Geometry: final body of the model. Coordinates: model frame, mm. A direction names the side the tool comes from. Round coordinates to 2 decimals unless told otherwise and drop trailing zeros. Loops run counter-clockwise (first coordinate to the right, second up) from the corner with the lowest first, then second, coordinate; pieces in that order, holes last. Notation, with made-up numbers: M -6.5,41.5 L 37.5,41.5 A18 ccw 37.5,61.5 Z; hole C -33.75,19 d5. An arc over 180 degrees is marked long. Answer as a JSON object with one key per item and string values.
```python
from build123d import *

# Parameters (mm, degrees)
SKETCH1_R             = 25
BOSS_EXTRUDE1_DEPTH   = 8
CUT_EXTRUDE1_DEPTH    = 2
CUT_EXTRUDE2_DEPTH    = 36.860842154
M3X0_5_TAPPED_HOLE1_D = 2.5
CUT_EXTRUDE3_DEPTH    = 37.249137921
SKETCH7_W             = 20
SKETCH7_H             = 6
CUT_EXTRUDE4_DEPTH    = 37.249137921
FILLET1_R             = 1.5


with BuildPart() as part:
    # Sketch1 → Boss-Extrude1 (new body)
    with BuildSketch(Plane.XY):
        Circle(SKETCH1_R)
    extrude(amount=-BOSS_EXTRUDE1_DEPTH)

    # Sketch2 → Cut-Extrude1 (cut)
    with BuildSketch(Plane.XY):
        with BuildLine():
            Line((-17.5, 12.5), (17.5, 12.5))
            ThreePointArc((17.5, 12.5), (19.267766953, 11.767766953), (20, 10))
            Line((20, 10), (20, -10))
            ThreePointArc((20, -10), (19.267766953, -11.767766953), (17.5, -12.5))
            Line((17.5, -12.5), (-17.5, -12.5))
            ThreePointArc((-17.5, -12.5), (-19.267766953, -11.767766953), (-20, -10))
            Line((-20, -10), (-20, 10))
            ThreePointArc((-20, 10), (-19.267766953, 11.767766953), (-17.5, 12.5))
        make_face()
    extrude(amount=-CUT_EXTRUDE1_DEPTH, mode=Mode.SUBTRACT)

    # Sketch3 → Cut-Extrude2 (cut, through all)
    with BuildSketch(Plane.XY.offset(-2)):
        with BuildLine():
            Line((-7.5, 5), (7.5, 5))
            ThreePointArc((7.5, 5), (12.5, 0), (7.5, -5))
            Line((7.5, -5), (-7.5, -5))
            ThreePointArc((-7.5, -5), (-12.5, 0), (-7.5, 5))
        make_face()
    extrude(amount=-CUT_EXTRUDE2_DEPTH, mode=Mode.SUBTRACT)

    # M3x0.5 Tapped Hole1 (through all)
    with Locations(Plane.XY.offset(-2)):
        with Locations((16, 8.5), (-16, 8.5), (-16, -8.5), (16, -8.5)):
            Hole(M3X0_5_TAPPED_HOLE1_D / 2)

    # Sketch6 → Cut-Extrude3 (cut, through all)
    with BuildSketch(Plane.XY):
        with BuildLine():
            Line((6, 21.75), (-6, 21.75))
            ThreePointArc((-6, 21.75), (-7.060660172, 21.310660172), (-7.5, 20.25))
            Line((-7.5, 20.25), (-7.5, 15.75))
            ThreePointArc((-7.5, 15.75), (-7.060660172, 14.689339828), (-6, 14.25))
            Line((-6, 14.25), (6, 14.25))
            ThreePointArc((6, 14.25), (7.060660172, 14.689339828), (7.5, 15.75))
            Line((7.5, 15.75), (7.5, 20.25))
            ThreePointArc((7.5, 20.25), (7.060660172, 21.310660172), (6, 21.75))
        make_face()
    extrude(amount=-CUT_EXTRUDE3_DEPTH, mode=Mode.SUBTRACT)

    # Sketch7 → Cut-Extrude4 (cut, through all)
    with BuildSketch(Plane.XY):
        with Locations((0, -18)):
            Rectangle(SKETCH7_W, SKETCH7_H)
    extrude(amount=-CUT_EXTRUDE4_DEPTH, mode=Mode.SUBTRACT)

    # Fillet1
    fillet1_edges = [part.edges().sort_by_distance(p)[0] for p in [
        (10, -15, -4),
        (10, -21, -4),
        (-10, -21, -4),
        (-10, -15, -4),
    ]]
    fillet(fillet1_edges, radius=FILLET1_R)


solid = part.part
```
1) Cut plane A-A on y = 0. Return the cut outline in (x, z).
Geometry results:
{"outline": "M -25,-8 L -12.5,-8 L -12.5,-2 L -20,-2 L -20,0 L -25,0 Z; M 12.5,-8 L 25,-8 L 25,0 L 20,0 L 20,-2 L 12.5,-2 Z"}
2) Set-up query: faces 3 (the face through (20, 0, -1)), 4 (the face through (-0.3, -5.2, -8)), 5 (the face through (0, 5, -5)). Return all of +Z, -Z, +X, -X, +Y, -Y with unobstructed straight access to the full face (end or side cutting, diameter ignored); none if empty.
Geometry results:
{"face 3": "+Z", "face 4": "-Z, +X, -X, +Y, -Y", "face 5": "+Z, -Z"}
3) Pull-direction query (X, two-part tool) for faces 1 (the face through (10, -18, -4)), 2 (the face through (0, 13, 0)); classes: +X half, -X half, draft (parallel to the pull), parting line (faces both ways), or undercut.
Geometry results:
{"face 1": "undercut", "face 2": "draft"}
4) Line query: probe 1 along Y at (x, z) = (-2.5, -1.5); probe 2 along Z at (x, y) = (0, -7.5); probe 3 along Y at (x, z) = (8.5, -0.75). Output: solid intervals per line, ascending.
Geometry results:
{"probe 1": "-24.87 to -21, -15 to -12.5, 12.5 to 14.25, 21.75 to 24.87", "probe 2": "-8 to -2", "probe 3": "-23.51 to -21, -15 to -12.5, 12.5 to 23.51"}
5) First-contact query: pin 1 (1 mm diameter, centred on x = 3, z = -1.5, fed in from -Y); pin 2 (4 mm diameter, centred on x = -2, z = -4.5, fed in from -Y); pin 3 (2 mm diameter, centred on y = 13.5, z = -4.5, fed in from +X). Flat tips, straight axial feed; report the tip coordinate or a pass-through.
Geometry results:
{"pin 1": "y = -24.87", "pin 2": "y = -25", "pin 3": "x = 21.65"}
6) Cut plane B-B on z = -4.5. Return the cut outline in (x, y), and give its area (3 significant figures).
Geometry results:
{"outline": "C 0,0 d50; hole C -16,-8.5 d2.5; hole C -16,8.5 d2.5; hole M -10,-19.5 A1.5 ccw -8.5,-21 L 8.5,-21 A1.5 ccw 10,-19.5 L 10,-16.5 A1.5 ccw 8.5,-15 L -8.5,-15 A1.5 ccw -10,-16.5 Z; hole M -7.5,-5 L 7.5,-5 A5 ccw 7.5,5 L -7.5,5 A5 ccw Z; hole M -7.5,15.75 A1.5 ccw -6,14.25 L 6,14.25 A1.5 ccw 7.5,15.75 L 7.5,20.25 A1.5 ccw 6,21.75 L -6,21.75 A1.5 ccw -7.5,20.25 Z; hole C 16,-8.5 d2.5; hole C 16,8.5 d2.5", "area": "1,490 mm2"}
7) Cut plane C-C on z = -1. Return the cut outline in (x, y), and give its area (3 significant figures).
Geometry results:
{"outline": "C 0,0 d50; hole M -20,-10 A2.5 ccw -17.5,-12.5 L 17.5,-12.5 A2.5 ccw 20,-10 L 20,10 A2.5 ccw 17.5,12.5 L -17.5,12.5 A2.5 ccw -20,10 Z; hole M -10,-19.5 A1.5 ccw -8.5,-21 L 8.5,-21 A1.5 ccw 10,-19.5 L 10,-16.5 A1.5 ccw 8.5,-15 L -8.5,-15 A1.5 ccw -10,-16.5 Z; hole M -7.5,15.75 A1.5 ccw -6,14.25 L 6,14.25 A1.5 ccw 7.5,15.75 L 7.5,20.25 A1.5 ccw 6,21.75 L -6,21.75 A1.5 ccw -7.5,20.25 Z", "area": "740 mm2"}
8) Cut plane D-D on y = 8.5. Return the cut outline in (x, z), and give its area (3 significant figures).
Geometry results:
{"outline": "M -23.51,-8 L -17.25,-8 L -17.25,-2 L -20,-2 L -20,0 L -23.51,0 Z; M -14.75,-8 L 14.75,-8 L 14.75,-2 L -14.75,-2 Z; M 17.25,-8 L 23.51,-8 L 23.51,0 L 20,0 L 20,-2 L 17.25,-2 Z", "area": "266 mm2"}
